```python
from build123d import *

# Parameters (mm, degrees)
SKETCH1_R                 = 6.35
BOSS_EXTRUDE1_DEPTH       = 15.875
SKETCH2_R                 = 3.1
CUT_EXTRUDE1_DEPTH        = 9.525
SKETCH3_R                 = 4.1
CUT_EXTRUDE2_DEPTH        = 6.35
F_6_32_TAPPED_HOLE1_D     = 2.7051
F_6_32_TAPPED_HOLE1_DEPTH = 7
F_6_32_TAPPED_HOLE1_TIP   = 0.81269403
F_6_32_TAPPED_HOLE2_D     = 2.7051


with BuildPart() as part:
    # Sketch1 → Boss-Extrude1 (new body)
    with BuildSketch(Plane(origin=(0, 0, 0), x_dir=(0, 0, -1), z_dir=(0, -1, 0))):
        Circle(SKETCH1_R)
    extrude(amount=BOSS_EXTRUDE1_DEPTH)

    # Sketch2 → Cut-Extrude1 (cut)
    with BuildSketch(Plane(origin=(0, 0, 0), x_dir=(1, 0, 0), z_dir=(0, 1, 0))):
        Circle(SKETCH2_R)
    extrude(amount=-CUT_EXTRUDE1_DEPTH, mode=Mode.SUBTRACT)

    # Sketch3 → Cut-Extrude2 (cut)
    with BuildSketch(Plane.XZ.offset(15.875)):
        Circle(SKETCH3_R)
    extrude(amount=-CUT_EXTRUDE2_DEPTH, mode=Mode.SUBTRACT)

    # #6-32 Tapped Hole1
    with Locations(Plane(origin=(-6.349702391, -3.685069286, 0.061478042), x_dir=(-0.009681581, 0, -0.999953132), z_dir=(-0.999953132, 0, 0.009681581))):
        with Locations((0, 0)):
            Hole(F_6_32_TAPPED_HOLE1_D / 2, depth=F_6_32_TAPPED_HOLE1_DEPTH)
            with Locations((0, 0, -(F_6_32_TAPPED_HOLE1_DEPTH + F_6_32_TAPPED_HOLE1_TIP / 2))):  # 118° drill point
                Cone(0, F_6_32_TAPPED_HOLE1_D / 2, F_6_32_TAPPED_HOLE1_TIP, mode=Mode.SUBTRACT)

    # #6-32 Tapped Hole2 (through all)
    with Locations(Plane(origin=(-6.349688123, -12.545322132, 0.062934409), x_dir=(-0.009910931, 0, -0.999950886), z_dir=(-0.999950886, 0, 0.009910931))):
        with Locations((0, 0)):
            Hole(F_6_32_TAPPED_HOLE2_D / 2)


solid = part.part
```
For this review, take the finished solid that the model builds, in its own axes (mm). A direction names the side the tool comes from. Give positions to 0.01 mm unless a question says otherwise; leave off trailing zeros. Order: outer loops, then holes, each group sorted by start corner. A loop starts at its lowest first (then second) coordinate and runs counter-clockwise, first axis right, second up.
1) Take a section at C-C (y = -12.25). Give the boundary of the cut face in (x, z).
2) The part is to be moulded in two halves that separate along Y. For faces 1 (the face through (-2, -9.525, 3)), 2 (the face through (-5.1, -12.6, -1.3)), 3 (the face through (2, 0, -3)), say which applies: released by +Y, released by -Y, zero draft, split by the parting line, or undercut.
3) Take a section at B-B (y = -6). Give the boundary of the cut face in (x, z), then the cut area to 3 significant figures.
4) Take a section at A-A (x = 0). Give the boundary of the cut face in (y, z) (3 decimals).
5) Insertion check: pin 1 (3 mm diameter, centred on y = -11, z = -4.5, fed in from +X); pin 2 (2 mm diameter, centred on x = -4, y = -8, fed in from +Z). Each pin has a flat end and moves straight along its axis. Give the tip position at first contact, or say it passes through.
6) Wall thickness on line 1 (X direction, y = -14, z = 0); line 2 (X direction, y = -6.5, z = -1.25); line 3 (Y direction, x = -3.5, z = 1.75) (3 decimals): over which ranges is each line inside the solid? List them lowest first.
7) For faces 4 (the face through (-4.56, -3.745, -1.307)), 5 (the face through (3.787, -12.744, -1.57)), 6 (the face through (-4.1, -15.875, -1.3)), list the 3-axis set-ups (+Z, -Z, +X, -X, +Y, -Y) from which the entire face can be reached by the end or side of a thin tool; tool diameter is ignored.
8) Take a section at D-D (z = -0.5). State how many separate pieces and enclosed holes the cut face has, then the cut area to 3 significant figures.
Derived:
1. outline: (-6.22, -1.26) arc R6.35 ccw to (6.2, -1.38) - (3.87, -1.36) arc R4.1 cw to (-3.89, -1.28) - close; (-6.2, 1.38) - (-3.87, 1.36) arc R4.1 cw to (3.89, 1.28) - (6.22, 1.26) arc R6.35 ccw to start
2. face 1: released by -Y
2. face 2: undercut
2. face 3: released by +Y
3. outline: circle Ø12.7 at (0, 0); hole circle Ø6.2 at (0, 0)
3. area: 96.5 mm2
4. outline: (-15.875, -6.35) - (0, -6.35) - (0, -3.1) - (-9.525, -3.1) - (-9.525, -4.1) - (-15.875, -4.1) - close; (-15.875, 4.1) - (-9.525, 4.1) - (-9.525, 3.1) - (0, 3.1) - (0, 6.35) - (-15.875, 6.35) - close
5. pin 1: stops at x = 5.6
5. pin 2: stops at z = 5.6
6. line 1: x = -6.35 to -4.1, 4.1 to 6.35
6. line 2: x = -6.23 to -2.84, 2.84 to 6.23
6. line 3: y = -9.525 to 0
7. face 4: none
7. face 5: -Y
7. face 6: +Z, -Z, +X, -X, -Y
8. separate pieces: 5
8. enclosed holes: 0
8. area: 71.6 mm2
